Verification items for this drawing (mm, ordinates from the low corner). Round coordinates to 2 decimals unless told otherwise and drop trailing zeros. Order: outer loops, then holes, each group sorted by start corner. A loop starts at its lowest first (then second) coordinate and runs counter-clockwise, first axis right, second up. Notation, with made-up numbers: (37, 68.5) -> (60, 68.5) arc R27 ccw to (60, 89.5) -> close; hole circle Ø9 at (2, 85.5). An arc over 180 degrees is marked (long way). Answer in a Markdown table with one row per item.
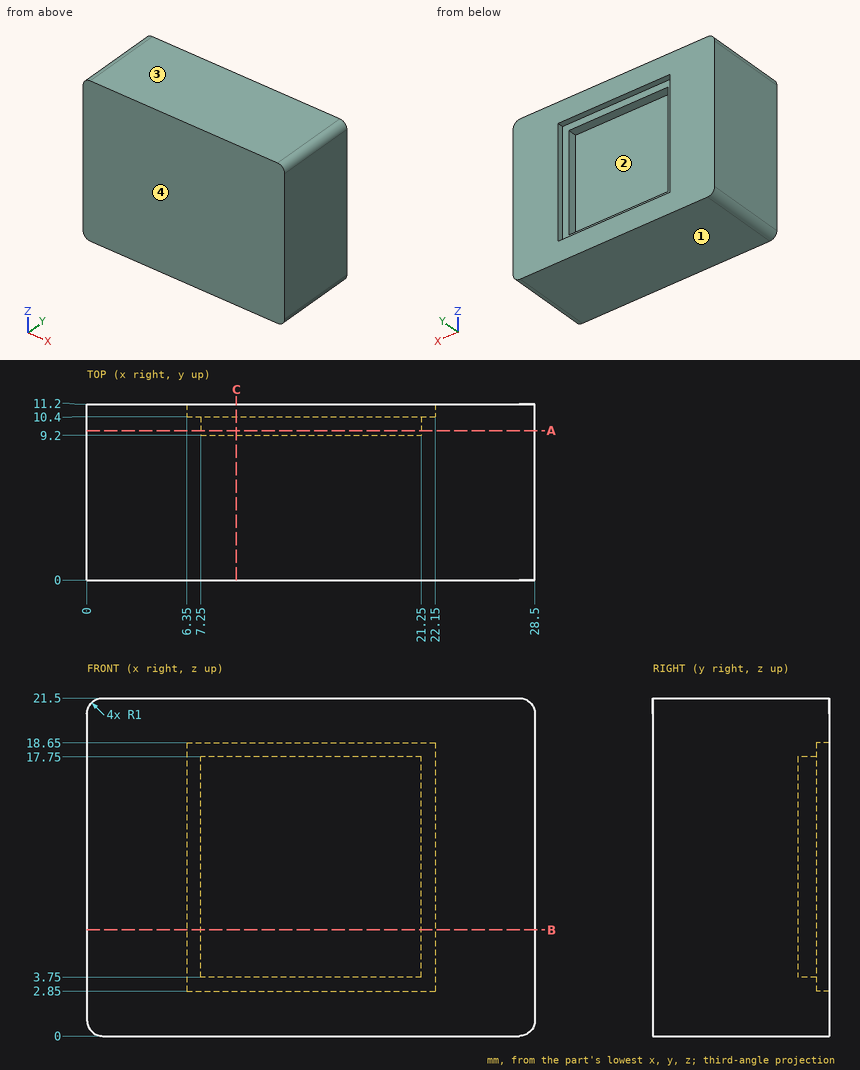
Item 1: Cross-section at A-A (y = 9.5). Record the boundary of the cut face in (x, z), and give its area (3 significant figures).
Result sheet:
| item | result |
|---|---|
| outline | (0, 1) arc R1 ccw to (1, 0) -> (27.5, 0) arc R1 ccw to (28.5, 1) -> (28.5, 20.5) arc R1 ccw to (27.5, 21.5) -> (1, 21.5) arc R1 ccw to (0, 20.5) -> close; hole (7.25, 3.75) -> (21.25, 3.75) -> (21.25, 17.75) -> (7.25, 17.75) -> close |
| area | 416 mm^2 |
Item 2: Depth check by flat-ended pin: P1, Ø4, axis at x = 14, z = 14, coming from the +Y side; P2, Ø2, axis at x = 21, z = 16.5, coming from the -Y side; P3, Ø8, axis at x = 10.5, z = 7, coming from the +Y side. Enter the tip coordinate at first touch or a pass-through.
Result sheet:
| item | result |
|---|---|
| P1 | stops at y = 9.2 |
| P2 | stops at y = 0 |
| P3 | stops at y = 10.4 |
Item 3: Cross-section at B-B (z = 6.75). Record the boundary of the cut face in (x, y), and give its area (3 significant figures).
Result sheet:
| item | result |
|---|---|
| outline | (0, 0) -> (28.5, 0) -> (28.5, 11.2) -> (22.15, 11.2) -> (22.15, 10.4) -> (21.25, 10.4) -> (21.25, 9.2) -> (7.25, 9.2) -> (7.25, 10.4) -> (6.35, 10.4) -> (6.35, 11.2) -> (0, 11.2) -> close |
| area | 290 mm^2 |
Item 4: Cross-section at C-C (x = 9.5). Record the boundary of the cut face in (y, z), and give its area (3 significant figures).
Result sheet:
| item | result |
|---|---|
| outline | (0, 0) -> (11.2, 0) -> (11.2, 2.85) -> (10.4, 2.85) -> (10.4, 3.75) -> (9.2, 3.75) -> (9.2, 17.75) -> (10.4, 17.75) -> (10.4, 18.65) -> (11.2, 18.65) -> (11.2, 21.5) -> (0, 21.5) -> close |
| area | 211 mm^2 |
Item 5: Scan lines: line 1 (X direction, y = 10.25, z = 10.5); line 2 (Z direction, x = 16.25, y = 10.25); line 3 (Y direction, x = 17.5, z = 12.5). Record each from-to range of solid material in increasing order. Write a range as [from, to].
Result sheet:
| item | result |
|---|---|
| line 1 | x = [0, 7.25], [21.25, 28.5] |
| line 2 | z = [0, 3.75], [17.75, 21.5] |
| line 3 | y = [0, 9.2] |
Item 6: Mould release check, pull along Z, two halves, no side actions. Record for the marked faces 1, 2, 3 and 4: pulls with the +Z half, pulls with the -Z half, needs draft (parallel to the pull), parting line crosses it, or undercut.
Result sheet:
| item | result |
|---|---|
| face 1 | pulls with the -Z half |
| face 2 | undercut |
| face 3 | pulls with the +Z half |
| face 4 | needs draft |
